For this review, take the finished solid that the model builds, in its own axes (mm). A direction names the side the tool comes from. Round coordinates to 2 decimals unless told otherwise and drop trailing zeros. Loops run counter-clockwise (first coordinate to the right, second up) from the corner with the lowest first, then second, coordinate; pieces in that order, holes last.
1) Take a section at B-B (y = 21.5). State the section outline as (x, z) points.
2) Wall thickness on L1, parallel to Y at x = 17.5, z = 5.5; L2, parallel to X at y = 25.5, z = 8.75; L3, parallel to Y at x = 62, z = 5.75: over which ranges is each line inside the solid? List them lowest first.
3) Take a section at C-C (y = 10). State the section outline as (x, z) points, then the cut area to 3 significant figures.
4) Mouldability with a two-part tool opening along X and no side actions: class faces 3 (the flat face through (70, 18, 0)), 4 (the flat face through (116, 17, 5)), 5 (the flat face through (42, 20, 6)) as pulls with the +X half, pulls with the -X half, needs draft (parallel to the pull), parting line crosses it, or undercut.
5) Take a section at D-D (z = 7.5). Give the number of separate pieces and of enclosed holes in the cut face, then the cut area to 3 significant figures.
6) Tool access review of faces 1 (the cylindrical face through (80, 28, 4)), 2 (the flat face through (65, 35, 5)): name each direction out of +Z, -Z, +X, -X, +Y, -Y from which nothing blocks a thin tool from reaching the whole face with its end or side.
7) Take a section at A-A (x = 61). State the section outline as (y, z) points, then the cut area to 3 significant figures.
```python
from build123d import *

# Parameters (mm, degrees)
F0_R     = 12.5
F1_DEPTH = 10


with BuildPart() as f1:
    # F0 (on Top) → F1 (new body)
    with BuildSketch(Plane.XY):
        with BuildLine():
            ThreePointArc((0, 17.5), (5.1256313292, 5.1256313292), (17.5, 0))
            Line((17.5, 0), (111, 0))
            ThreePointArc((111, 0), (114.5355339059, 1.4644660941), (116, 5))
            Line((116, 5), (116, 30))
            ThreePointArc((116, 30), (114.5355339059, 33.5355339059), (111, 35))
            Line((111, 35), (17.5, 35))
            ThreePointArc((17.5, 35), (5.1256313292, 29.8743686708), (0, 17.5))
        make_face()
        with Locations((17.5, 17.5)):
            Circle(F0_R, mode=Mode.SUBTRACT)
    extrude(amount=F1_DEPTH)

    # F2 (on face) → F3 (revolve, cut)
    with BuildSketch(Plane.XY.offset(10)):
        Polygon((42, 20), (42, 6), (45.5, 6), (45.5, 20), (49, 20), (49, 26), (48, 26), (48, 30), (42, 30), (42, 26), align=None)
    revolve(axis=Axis((42, 13, 10), (0, 1, 0)), mode=Mode.SUBTRACT)

    # F2 (on face) → F4 (revolve, cut)
    with BuildSketch(Plane.XY.offset(10)):
        Polygon((61, 20), (61, 6), (64.5, 6), (64.5, 20), (68, 20), (68, 26), (67, 26), (67, 30), (61, 30), (61, 26), align=None)
    revolve(axis=Axis((61, 13, 10), (0, 1, 0)), mode=Mode.SUBTRACT)

    # F2 (on face) → F5 (revolve, cut)
    with BuildSketch(Plane.XY.offset(10)):
        Polygon((80, 20), (80, 6), (83.5, 6), (83.5, 20), (87, 20), (87, 26), (86, 26), (86, 30), (80, 30), (80, 26), align=None)
    revolve(axis=Axis((80, 13, 10), (0, 1, 0)), mode=Mode.SUBTRACT)

    # F7 (on offset) → F8 (revolve, cut)
    with BuildSketch(Plane.XY.offset(11)):
        Polygon((101.5, 19), (101.5, 3), (106, 3), (106, 19), (111, 19), (111, 26.5), (108.5, 26.5), (108.5, 31.5), (101.5, 31.5), (101.5, 26.5), align=None)
    revolve(axis=Axis((101.5, 11, 11), (0, 1, 0)), mode=Mode.SUBTRACT)


solid = f1.part
```
Response:
1. outline: (0.46, 0) - (5.66, 0) - (5.66, 10) - (0.46, 10) - close; (29.34, 0) - (116, 0) - (116, 10) - (110.95, 10) arc R9.5 cw to (92.05, 10) - (87, 10) arc R7 cw to (73, 10) - (68, 10) arc R7 cw to (54, 10) - (49, 10) arc R7 cw to (35, 10) - (29.34, 10) - close
2. L1: y = 0 to 5, 30 to 35
2. L2: x = 1.94 to 7.9, 27.1 to 35.11, 48.89 to 54.11, 67.89 to 73.11, 86.89 to 92.27, 110.73 to 116
2. L3: y = 0 to 20, 30 to 35
3. outline: (1.69, 0) - (7.5, 0) - (7.5, 10) - (1.69, 10) - close; (27.5, 0) - (116, 0) - (116, 10) - (105.89, 10) arc R4.5 cw to (97.11, 10) - (83.5, 10) arc R3.5 cw to (76.5, 10) - (64.5, 10) arc R3.5 cw to (57.5, 10) - (45.5, 10) arc R3.5 cw to (38.5, 10) - (27.5, 10) - close
3. area: 863 mm2
4. face 3: needs draft
4. face 4: pulls with the +X half
4. face 5: undercut
5. separate pieces: 1
5. enclosed holes: 5
5. area: 2,570 mm2
6. face 1: +Z
6. face 2: +Z, -Z, +X, -X, +Y
7. outline: (0, 0) - (35, 0) - (35, 10) - (30, 10) - (30, 4) - (26, 4) - (26, 3) - (20, 3) - (20, 6.5) - (6, 6.5) - (6, 10) - (0, 10) - close
7. area: 235 mm2
